Geometry: final body of the model. Coordinates: model frame, mm. Face numbers are marked on the shaded views. A direction names the side the tool comes from. Give positions to 0.01 mm unless a question says otherwise; leave off trailing zeros. Order: outer loops, then holes, each group sorted by start corner. A loop starts at its lowest first (then second) coordinate and runs counter-clockwise, first axis right, second up. Notation, with made-up numbers: M 70.25,27.5 L 86.25,27.5 A16 ccw 86.25,48.5 Z; hole C 21,-4 d5. An arc over 180 degrees is marked long. Write item = value, one per line. Start each with the question number.
from build123d import *

# Parameters (mm, degrees)
F2_SIZE  = 0.5
F3_W     = 18
F3_H     = 5
F4_DEPTH = 4.001
F5_R     = 1.5
F6_DEPTH = 5.1428832774
F7_R     = 1.5
F8_DEPTH = 4.0010001


with BuildPart() as f1:
    # F0 (on Right) → F1 (revolve)
    with BuildSketch(Plane.YZ):
        Polygon((0, 9), (0, 8), (3, 8), (3, 15), (-1, 15), (-1, 9), align=None)
    revolve(axis=Axis((0, 22.7407575149, 0), (0, 1, 0)))

    # F2
    f2_edges = [f1.edges().sort_by_distance(p)[0] for p in [
        (0, 3, -15),
        (0, -1, -15),
    ]]
    chamfer(f2_edges, length=F2_SIZE)

    # F3 (on face) → F4 (cut, through all)
    with BuildSketch(Plane.XZ.offset(1)):
        with Locations((0, -15.5)):
            Rectangle(F3_W, F3_H)
    extrude(amount=-F4_DEPTH, mode=Mode.SUBTRACT)

    # F5 (on face) → F6 (cut, through all)
    with BuildSketch(Plane(origin=(0, 0, -13), x_dir=(1, 0, 0), z_dir=(0, 0, -1))):
        with Locations((0, -1)):
            Circle(F5_R)
    extrude(amount=-F6_DEPTH, mode=Mode.SUBTRACT)

    # F7 (on face) → F8 (cut, through all)
    with BuildSketch(Plane.XZ.offset(1)):
        with Locations((0, 11.5)):
            Circle(F7_R)
        with Locations((-9.9592921435, -5.75)):
            Circle(F7_R)
        with Locations((9.9592921435, -5.75)):
            Circle(F7_R)
    extrude(amount=-F8_DEPTH, mode=Mode.SUBTRACT)


solid = f1.part
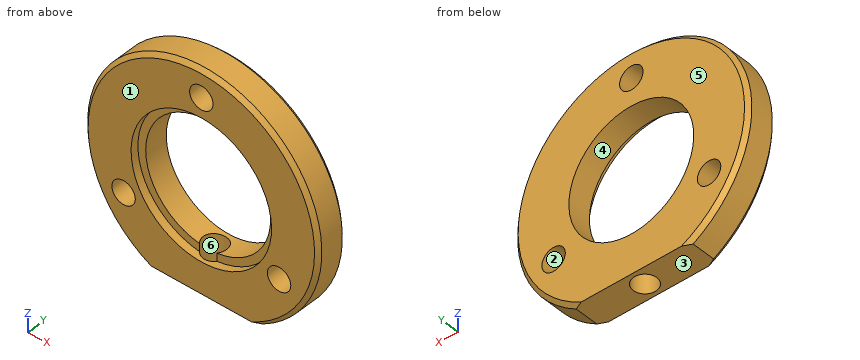
1) Ray query, L1, parallel to X at y = -0.35, z = 0; L2, parallel to Y at x = 0, z = -11.8; L3, parallel to Z at x = 0, y = 0.05. Return the intervals inside material, ascending.
2) Cut plane B-B (x = 0.75). Give the number of separate pieces and of enclosed holes in the cut face, plus the area to 3 significant figures.
3) Pin query (flat end, axial travel): pin 1 Ø3 at (x, z) = (-9, -5) entering from +Y; pin 2 Ø2.5 at (x, z) = (-9.96, -5.75) entering from +Y; pin 3 Ø1 at (y, z) = (1.5, -10) entering from +X; pin 4 Ø2 at (x, y) = (6, 2) entering from +Z. Return the tip coordinate at first contact, or that it passes through.
4) Access query for the marked faces 5 and 6. Directions: +Z, -Z, +X, -X, +Y, -Y. A direction counts if a zero-diameter tool reaches every point of the face in a straight line with its end or side. Return the directions, or none.
5) Draft query along Z for the marked faces 1, 2, 3 and 4. Return one class per face: pulls with the +Z half, pulls with the -Z half, needs draft (parallel to the pull), parting line crosses it, or undercut.
6) Cut plane A-A (y = 1). Return loops of the section in (x, z), plus the area to 3 significant figures.
Reply:
q1.L1 = -15 to -9, 9 to 15
q1.L2 = -1 to -0.5, 2.5 to 3
q1.L3 = 8 to 10, 13 to 15
q2.separate_pieces = 4
q2.enclosed_holes = 0
q2.area = 22.8 mm²
q3.pin_1 = 3
q3.pin_2 = through
q3.pin_3 = 11.61
q3.pin_4 = 14.14
q4.face_5 = +Z, -Z, +X, -X, +Y
q4.face_6 = -Z
q5.face_1 = needs draft
q5.face_2 = undercut
q5.face_3 = pulls with the -Z half
q5.face_4 = undercut
q6.outline = M -7.48,-13 L -1.5,-13 L -1.5,-7.86 A8 cw long 1.5,-7.86 L 1.5,-13 L 7.48,-13 A15 ccw long Z; hole C -9.96,-5.75 d3; hole C 0,11.5 d3; hole C 9.96,-5.75 d3
q6.area = 449 mm²
